Study the drawing (mm; zero at the part's minimum x, y, z) and answer. Round coordinates to 2 decimals unless told otherwise and drop trailing zeros. Order: outer loops, then holes, each group sorted by start corner. A loop starts at its lowest first (then second) coordinate and runs counter-clockwise, first axis right, second up. Notation, with made-up numbers: M -22,-19.75 L 28,-19.75 A10 ccw 28,-11.75 Z; hole C -32,86 d8. An arc over 180 degrees is marked long. Put each result on its own line as item: value. Start each with the question number.
1. Consider line 1 (Z direction, x = 64, y = 0.5); line 2 (X direction, y = 1.5, z = 52); line 3 (Z direction, x = 9, y = 0.6). Determine where each line is inside the solid, lowest interval first.
2. The part is cut by section A-A (z = 52). Give the vertices of the cut face in (x, y), then the cut area to 3 significant figures.
3. The part is cut by section B-B (x = 64). Give the vertices of the cut face in (y, z), then the cut area to 3 significant figures.
4. The part is cut by section C-C (x = 9). Give the vertices of the cut face in (y, z), then the cut area to 3 significant figures.
5. The part is cut by section D-D (y = 0.7). Give the vertices of the cut face in (x, z).
6. This flat-tipped pin is pushed along its axis until it touches: pin 1 Ø0.6 at (y, z) = (1, 35.5) entering from -X. Where does it stop, or does it pass through?
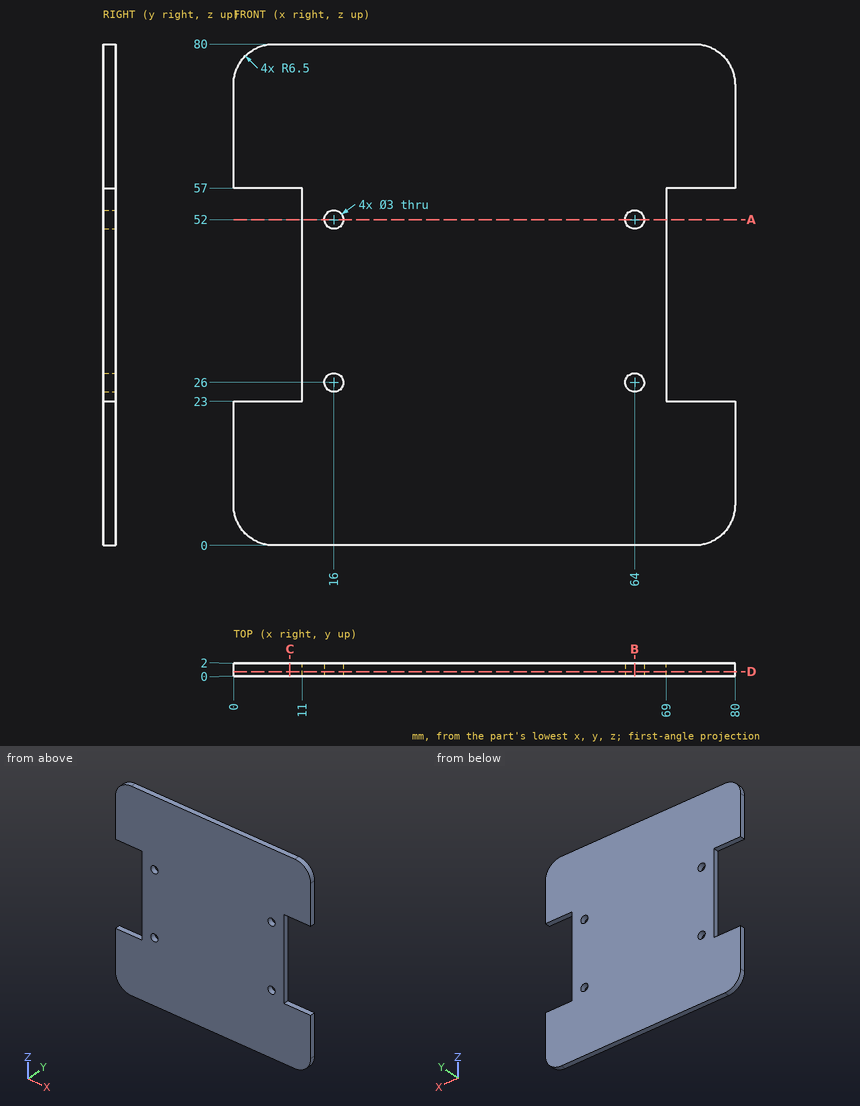
Resolved:
1. line 1: 0 to 24.5, 27.5 to 50.5, 53.5 to 80
1. line 2: 11 to 14.5, 17.5 to 62.5, 65.5 to 69
1. line 3: 0 to 23, 57 to 80
2. outline: M 11,0 L 14.5,0 L 14.5,2 L 11,2 Z; M 17.5,0 L 62.5,0 L 62.5,2 L 17.5,2 Z; M 65.5,0 L 69,0 L 69,2 L 65.5,2 Z
2. area: 104 mm2
3. outline: M 0,0 L 2,0 L 2,24.5 L 0,24.5 Z; M 0,27.5 L 2,27.5 L 2,50.5 L 0,50.5 Z; M 0,53.5 L 2,53.5 L 2,80 L 0,80 Z
3. area: 148 mm2
4. outline: M 0,0 L 2,0 L 2,23 L 0,23 Z; M 0,57 L 2,57 L 2,80 L 0,80 Z
4. area: 92.0 mm2
5. outline: M 0,6.5 A6.5 ccw 6.5,0 L 73.5,0 A6.5 ccw 80,6.5 L 80,23 L 69,23 L 69,57 L 80,57 L 80,73.5 A6.5 ccw 73.5,80 L 6.5,80 A6.5 ccw 0,73.5 L 0,57 L 11,57 L 11,23 L 0,23 Z; hole C 16,26 d3; hole C 16,52 d3; hole C 64,26 d3; hole C 64,52 d3
6. pin 1: x = 11
